```python
from build123d import *

# Parameters (mm, degrees)
SKETCH1_W                = 20.4
SKETCH1_H                = 18.9
BOSS_EXTRUDE1_DEPTH      = 3
M3_CLEARANCE_HOLE1_D     = 3.6
SKETCH4_W                = 20.4
SKETCH4_H                = 2.4
BOSS_EXTRUDE2_DEPTH      = 1.5
BOSS_EXTRUDE3_DEPTH      = 4
BOSS_EXTRUDE3_DEPTH_BACK = 0.1
SKETCH5_W                = 20.4
SKETCH5_H                = 9.3
CHAMFER1_SIZE            = 3.6
CHAMFER1_SIZE2           = 2.6
FILLET2_R                = 1
CHAMFER3_SIZE            = 1
FILLET1_R                = 0.6
RIB1_REACH               = 31.427
SKETCH7_WALL_W           = 68.853377202
SKETCH7_WALL_H           = 2
RIB2_START               = -1.5
RIB2_DEPTH               = 1.5
RIB10_REACH              = 36.323
SKETCH9_WALL_W           = 78.645466102
SKETCH9_WALL_H           = 1.5


# Read off the part's stored shape, not the designer's step: Rib2
with BuildPart() as part:
    # Sketch1 → Boss-Extrude1 (new body)
    with BuildSketch(Plane(origin=(0, 0, 0), x_dir=(1, 0, 0), z_dir=(0, 1, 0))):
        with Locations((10.2, 9.45)):
            Rectangle(SKETCH1_W, SKETCH1_H)
    extrude(amount=BOSS_EXTRUDE1_DEPTH)

    # M3 Clearance Hole1 (through all)
    with Locations(Plane(origin=(0, 3, 0), x_dir=(1, 0, 0), z_dir=(0, 1, 0))):
        with Locations((5.2, 4.2), (5.2, 14.2), (15.2, 14.2), (15.2, 4.2)):
            Hole(M3_CLEARANCE_HOLE1_D / 2)

    # Sketch4 → Boss-Extrude2 (add)
    with BuildSketch(Plane(origin=(0, 0, -18.9), x_dir=(-1, 0, 0), z_dir=(0, 0, -1))):
        with Locations((-10.2, 1.2)):
            Rectangle(SKETCH4_W, SKETCH4_H)
    extrude(amount=-BOSS_EXTRUDE2_DEPTH)

    # Sketch5 → Boss-Extrude3 (add, two sides: drawn at the far end of the back side and taken through both)
    with BuildSketch(Plane(origin=(0, 3, 0), x_dir=(1, 0, 0), z_dir=(0, 1, 0)).offset(-BOSS_EXTRUDE3_DEPTH_BACK)):
        with Locations((10.2, 22.05)):
            Rectangle(SKETCH5_W, SKETCH5_H)
    extrude(amount=BOSS_EXTRUDE3_DEPTH + BOSS_EXTRUDE3_DEPTH_BACK)

    # Chamfer1
    chamfer1_edges = [part.edges().sort_by_distance(p)[0] for p in [
        (20.4, 2.9, -22.8),
        (0, 2.9, -22.8),
    ]]
    chamfer1_side = [part.faces().sort_by_distance(p)[0] for p in [
        (10.2, 2.9, -22.8),
    ]]
    chamfer(chamfer1_edges, length=CHAMFER1_SIZE, length2=CHAMFER1_SIZE2, reference=chamfer1_side[0])

    # Fillet2
    fillet2_edges = [part.edges().sort_by_distance(p)[0] for p in [
        (20.4, 5.5, -22.8),
        (3.6, 2.9, -22.8),
        (16.8, 2.9, -22.8),
        (0, 5.5, -22.8),
    ]]
    fillet(fillet2_edges, radius=FILLET2_R)

    # Chamfer3
    chamfer3_edges = [part.edges().sort_by_distance(p)[0] for p in [
        (16.784315179, 2.94850664, -26.7),
        (20.290362441, 5.556058922, -26.7),
        (20.4, 6.505655648, -26.7),
        (18.523813503, 4.144976419, -26.7),
        (10.2, 2.9, -26.7),
        (1.876186497, 4.144976419, -26.7),
        (0, 6.505655648, -26.7),
        (0.109637559, 5.556058922, -26.7),
        (3.615684821, 2.94850664, -26.7),
    ]]
    chamfer(chamfer3_edges, length=CHAMFER3_SIZE - 0.0001)  # a hair under: the kernel refuses the full size

    # Fillet1
    fillet1_edges = [part.edges().sort_by_distance(p)[0] for p in [
        (0, 1.5, 0),
        (20.4, 1.5, 0),
        (20.4, 3.005655648, -18.9),
        (0, 3.005655648, -18.9),
    ]]
    fillet(fillet1_edges, radius=FILLET1_R)

    # Sketch7 wall → Rib1 (add, up to next)
    with BuildSketch(Plane(origin=(10.2, 5, -13.935898385), x_dir=(0, -0.500000000015, 0.866025403776), z_dir=(0, 0.866025403776, 0.500000000015)), mode=Mode.PRIVATE) as rib1_sk1:
        Rectangle(SKETCH7_WALL_W, SKETCH7_WALL_H)
    rib1_tool1 = extrude(rib1_sk1.sketch, amount=-RIB1_REACH, mode=Mode.PRIVATE) - part.part
    add(rib1_tool1.solids().sort_by_distance((10.2, 5, -13.935898385))[0])

    # Rib2 outline → Rib2 (add)
    with BuildSketch(Plane.ZY.offset(RIB2_START)):
        Polygon((-10.47179677, 3), (-17.4, 7), (-17.4, 3), align=None)
    extrude(amount=RIB2_DEPTH)

    # Sketch9 wall → Rib10 (add, up to next)
    with BuildSketch(Plane(origin=(20.4, 5, -13.935898385), x_dir=(0, -0.500000000015, 0.866025403776), z_dir=(0, -0.866025403776, -0.500000000015)), mode=Mode.PRIVATE) as rib10_sk1:
        with Locations((0, 0.75)):
            Rectangle(SKETCH9_WALL_W, SKETCH9_WALL_H)
    rib10_tool1 = extrude(rib10_sk1.sketch, amount=RIB10_REACH, mode=Mode.PRIVATE) - part.part
    add(rib10_tool1.solids().sort_by_distance((20.4, 5, -13.935898385))[0])


solid = part.part
```
The listing builds one solid part. Answer for the finished solid, in the listing's coordinates (mm). A direction names the side the tool comes from. Round coordinates to 2 decimals unless told otherwise and drop trailing zeros. Write each loop counter-clockwise with the first axis right and the second up, starting at its lowest first coordinate (ties: lowest second). Pieces come first, ordered by that corner, then holes. Notation, with made-up numbers: (4.5, 32.25) -> (18.5, 32.25) arc R5 cw to (18.5, 36.25) -> close; hole circle Ø4 at (-40, -31.5). An arc over 180 degrees is marked (long way). Use CSV: the item, a comma, the result in double quotes. Start each with the question number.
(1) Which of the six approach directions +Z, -Z, +X, -X, +Y, -Y give full straight-line access (tool end or side, diameter ignored) to faces 4 (the face through (10, 2.9, -22)), 5 (the face through (10.214, 5.028, -13.984)), 6 (the face through (15, 5, -17.4))?
(2) Section B-B on y = 2 is taken. Give the vertices of the cut face in (x, z).
(3) The mould has two halves that part along X. Classify faces 1 (the face through (0.107, 5.562, -22.052)), 2 (the face through (10, 0, -10)), 3 (the face through (11.2, 5, -15)): released by +X, released by -X, zero draft, split by the parting line, or undercut.
(4) Consider L1, parallel to X at y = 5, z = -16.5; L2, parallel to X at y = 1.5, z = -14.2; L3, parallel to Z at x = 5.2, y = 2.1. Determine where each line is inside the solid, lowest interval first. Write a range as from..to.
(5) Each of these flat-tipped pins is pushed along its axis until it touches: pin 1 (2 mm diameter, centred on x = 4.5, y = 5, fed in from +Z); pin 2 (4 mm diameter, centred on x = 12, z = -22.5, fed in from -Y); pin 3 (4.5 mm diameter, centred on x = 15.2, z = -4.2, fed in from +Y). Where does it stop, or does it pass through?
(6) Section A-A on x = 5.2 is taken. Give the vertices of the cut face in (y, z).
(7) Section D-D on x = 12 is taken. Give the vertices of the cut face in (y, z), then the cut area to 3 significant figures.
(8) Section C-C on z = -4.2 is taken. Give the vertices of the cut face in (x, y).
A:
1,face 4,"-Z, +X, -X, -Y"
1,face 5,"+Z, +X, -X, +Y"
1,face 6,"+Z, +Y"
2,outline,"(0, -18.3) arc R0.6 ccw to (0.6, -18.9) -> (19.8, -18.9) arc R0.6 ccw to (20.4, -18.3) -> (20.4, -0.6) arc R0.6 ccw to (19.8, 0) -> (0.6, 0) arc R0.6 ccw to (0, -0.6) -> close; hole circle Ø3.6 at (5.2, -14.2); hole circle Ø3.6 at (5.2, -4.2); hole circle Ø3.6 at (15.2, -14.2); hole circle Ø3.6 at (15.2, -4.2)"
3,face 1,"released by -X"
3,face 2,"zero draft"
3,face 3,"undercut"
4,L1,"x = 0..1.5, 9.2..11.2, 18.9..20.4"
4,L2,"x = 0..3.4, 7..13.4, 17..20.4"
4,L3,"z = -18.9..-16, -12.4..-6, -2.4..0"
5,pin 1,"stops at z = -17.4"
5,pin 2,"stops at y = 2.9"
5,pin 3,"stops at y = 3"
6,outline,"(0, -18.9) -> (2.9, -18.9) -> (2.9, -25.7) -> (3.9, -26.7) -> (7, -26.7) -> (7, -17.4) -> (3, -17.4) -> (3, -16) -> (0, -16) -> close; (0, -12.4) -> (3, -12.4) -> (3, -6) -> (0, -6) -> close; (0, -2.4) -> (3, -2.4) -> (3, 0) -> (0, 0) -> close"
7,outline,"(0, -18.9) -> (2.9, -18.9) -> (2.9, -25.7) -> (3.9, -26.7) -> (7, -26.7) -> (7, -17.4) -> (3, -17.4) -> (3, 0) -> (0, 0) -> close"
7,area,"94.2 mm²"
8,outline,"(0, 0) -> (3.4, 0) -> (3.4, 3) -> (0, 3) -> close; (7, 0) -> (13.4, 0) -> (13.4, 3) -> (7, 3) -> close; (17, 0) -> (20.4, 0) -> (20.4, 3) -> (17, 3) -> close"
